from build123d import *

# Parameters (mm, degrees)
F0_W     = 152.4
F0_H     = 101.6
F1_DEPTH = 50.8
F2_W     = 25.4
F2_H     = 76.2
F3_DEPTH = 50.8
F4_W     = 76.2
F4_H     = 50.8
F5_DEPTH = 50.801


with BuildPart() as f1:
    # F0 (on Top) → F1 (new body)
    with BuildSketch(Plane.XY):
        with Locations((76.2, -50.8)):
            Rectangle(F0_W, F0_H)
    extrude(amount=F1_DEPTH)

    # F2 (on face) → F3 (join)
    with BuildSketch(Plane.XY.offset(50.8)):
        with Locations((12.7, -38.1)):
            Rectangle(F2_W, F2_H)
    extrude(amount=F3_DEPTH)

    # F4 (on face) → F5 (cut, through all)
    with BuildSketch(Plane.XY.offset(50.8)):
        with Locations((114.3, -76.2)):
            Rectangle(F4_W, F4_H)
    extrude(amount=-F5_DEPTH, mode=Mode.SUBTRACT)


solid = f1.part
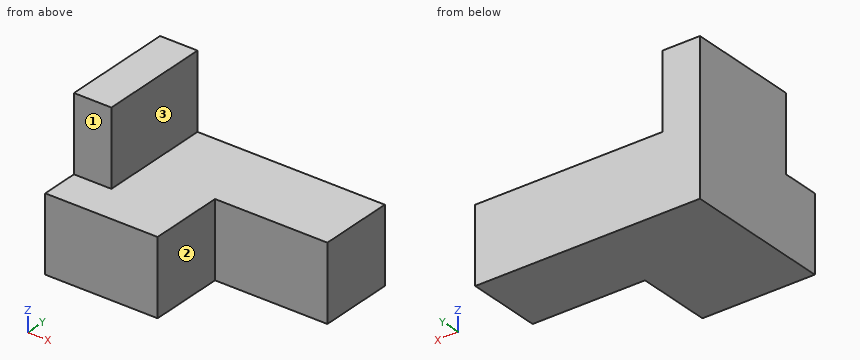
Design review of the part built by this model. Coordinates are the model's own, in mm. Face numbers are marked on the shaded views. A direction names the side the tool comes from. Coordinates: 2 decimals unless noted, no trailing zeros. Loops run counter-clockwise (first coordinate to the right, second up) from the corner with the lowest first, then second, coordinate; pieces in that order, holes last.
Item 1: For the marked faces 1, 2 and 3, list the 3-axis set-ups (+Z, -Z, +X, -X, +Y, -Y) from which the entire face can be reached by the end or side of a thin tool; tool diameter is ignored.
Completed:
face 1: +Z, +X, -X, -Y
face 2: +Z, -Z, +X, -Y
face 3: +Z, +X, +Y, -Y
Item 2: Add section B-B (z = 31.5). Write out the cut boundary in (x, y).
Completed:
outline: (0, -101.6) - (76.2, -101.6) - (76.2, -50.8) - (152.4, -50.8) - (152.4, 0) - (0, 0) - close
Item 3: Add section C-C (x = 34). Write out the cut boundary in (y, z), and give its area (3 significant figures).
Completed:
outline: (-101.6, 0) - (0, 0) - (0, 50.8) - (-101.6, 50.8) - close
area: 5,160 mm2
Item 4: Add section A-A (y = -73). Write out the cut boundary in (x, z), and give its area (3 significant figures).
Completed:
outline: (0, 0) - (76.2, 0) - (76.2, 50.8) - (25.4, 50.8) - (25.4, 101.6) - (0, 101.6) - close
area: 5,160 mm2
Item 5: Wall thickness on L1, parallel to X at y = -40, z = 97; L2, parallel to Z at x = 132, y = -38; L3, parallel to Y at x = 97.5, z = 31.5: over which ranges is each line inside the solid? List them lowest first.
Completed:
L1: x = 0 to 25.4
L2: z = 0 to 50.8
L3: y = -50.8 to 0
Item 6: Add section D-D (z = 72). Write out the cut boundary in (x, y), and give its area (3 significant figures).
Completed:
outline: (0, -76.2) - (25.4, -76.2) - (25.4, 0) - (0, 0) - close
area: 1,940 mm2
Item 7: Clearance check with flat-ended pins moving along their axes: pin 1 (20.5 mm diameter, centred on x = 7.5, z = 78, fed in from -Y); pin 2 (15 mm diameter, centred on x = 101.5, z = 22, fed in from -Y); pin 3 (2 mm diameter, centred on x = 85, y = -39, fed in from +Z). State where each tip first meets the part, or that it passes through.
Completed:
pin 1: stops at y = -76.2
pin 2: stops at y = -50.8
pin 3: stops at z = 50.8
